Input: part model. Units: mm. Frame: model coordinates. Face numbers are marked on the shaded views. A direction names the side the tool comes from. Round coordinates to 2 decimals unless told otherwise and drop trailing zeros. Loops run counter-clockwise (first coordinate to the right, second up) from the corner with the lowest first, then second, coordinate; pieces in that order, holes last. Notation, with made-up numbers: (21, 44) -> (44, 44) arc R24 ccw to (44, 58) -> close; hole circle Ø2 at (18.25, -11.75). An arc over 180 degrees is marked (long way). One line per question, with ' | ' between items. Start each with the question number.
Q1. Material intervals for L1, parallel to X at y = 1.1, z = 0; L2, parallel to X at y = 2.75, z = -2.5; L3, parallel to Z at x = 0, y = 0.95, sorted ascending.
Q2. Cut plane C-C on x = 12.5. Return loops of the section in (y, z) (3 decimals), and give its area (3 significant figures).
Q3. Contact query for flat-ended pins moving along their axis: P1, Ø0.8, axis at x = 14, z = 0, coming from the +Y side; P2, Ø5, axis at x = 11.6, z = 0, coming from the -Y side; P3, Ø3.5, axis at y = 2, z = 2, coming from the -X side; P4, Ø6, axis at x = 0.5, z = -1.5, coming from the -Y side. Output: stop coordinate, or through.
Q4. Mould query, pull axis X, two halves, no side actions, for the marked faces 1, 2, 3 and 4. Classes: pulls with the +X half, pulls with the -X half, needs draft (parallel to the pull), parting line crosses it, or undercut.
Q5. Access query for the marked faces 5, 6 and 7. Directions: +Z, -Z, +X, -X, +Y, -Y. A direction counts if a zero-diameter tool reaches every point of the face in a straight line with its end or side. Return the directions, or none.
Q6. Cut plane B-B on z = 0. Return loops of the section in (x, y).
Q7. Cut plane A-A on y = 0.75. Return loops of the section in (x, z), and give its area (3 significant figures).
Q8. Cut plane D-D on z = 3.25. Return loops of the section in (x, y).
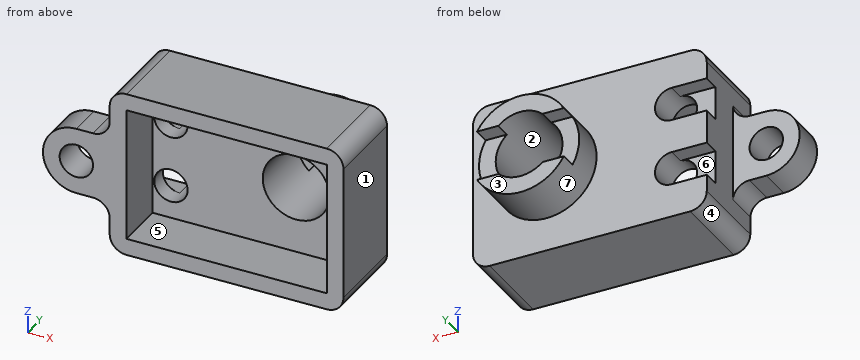
from build123d import *

# Parameters (mm, degrees)
SKETCH1_R           = 1
BOSS_EXTRUDE1_DEPTH = 5
SKETCH3_W           = 12
SKETCH3_H           = 8
CUT_EXTRUDE1_DEPTH  = 3
SKETCH4_R           = 3
SKETCH4_R_2         = 2
BOSS_EXTRUDE2_DEPTH = 3
SKETCH5_W           = 3
SKETCH5_H           = 1
CUT_EXTRUDE2_DEPTH  = 17
SKETCH6_R           = 2
SKETCH6_R_2         = 1
SKETCH6_W           = 7.064198251
SKETCH6_H           = 8.717344461
CUT_EXTRUDE3_DEPTH  = 6
CUT_EXTRUDE4_DEPTH  = 1


with BuildPart() as part:
    # Sketch1 → Boss-Extrude1 (new body)
    with BuildSketch(Plane(origin=(0, 0, 0), x_dir=(1, 0, 0), z_dir=(0, 1, 0))):
        with BuildLine():
            Line((1, 2), (0, 2))
            ThreePointArc((0, 2), (-2, 0), (0, -2))
            Line((0, -2), (1, -2))
            ThreePointArc((1, -2), (1.684527719, -2.270177533), (2, -2.935046948))
            Line((2, -2.935046948), (2, -4))
            ThreePointArc((2, -4), (2.292893219, -4.707106781), (3, -5))
            Line((3, -5), (15, -5))
            ThreePointArc((15, -5), (15.707106781, -4.707106781), (16, -4))
            Line((16, -4), (16, 4))
            ThreePointArc((16, 4), (15.707106781, 4.707106781), (15, 5))
            Line((15, 5), (3, 5))
            ThreePointArc((3, 5), (2.292893219, 4.707106781), (2, 4))
            Line((2, 4), (2, 2.932864189))
            ThreePointArc((2, 2.932864189), (1.684390871, 2.268771092), (1, 2))
        make_face()
        Circle(SKETCH1_R, mode=Mode.SUBTRACT)
    extrude(amount=BOSS_EXTRUDE1_DEPTH)

    # Sketch3 → Cut-Extrude1 (cut)
    with BuildSketch(Plane.XZ):
        with Locations((9, 0)):
            Rectangle(SKETCH3_W, SKETCH3_H)
    extrude(amount=-CUT_EXTRUDE1_DEPTH, mode=Mode.SUBTRACT)

    # Sketch4 → Boss-Extrude2 (add)
    with BuildSketch(Plane(origin=(0, 5, 0), x_dir=(1, 0, 0), z_dir=(0, 1, 0))):
        with Locations((11.597924937, 0)):
            Circle(SKETCH4_R)
        with Locations((11.597924937, 0)):
            Circle(SKETCH4_R_2, mode=Mode.SUBTRACT)
    extrude(amount=BOSS_EXTRUDE2_DEPTH)

    # Sketch5 → Cut-Extrude2 (cut)
    with BuildSketch(Plane.ZY.offset(-2)):
        with Locations((0, 7.5)):
            Rectangle(SKETCH5_W, SKETCH5_H)
    extrude(amount=-CUT_EXTRUDE2_DEPTH, mode=Mode.SUBTRACT)

    # Sketch6 → Cut-Extrude3 (cut)
    with BuildSketch(Plane(origin=(0, 8, 0), x_dir=(1, 0, 0), z_dir=(0, 1, 0))):
        with Locations((11.597924937, 0)):
            Circle(SKETCH6_R)
        with Locations((4.102933475, -2)):
            Circle(SKETCH6_R_2)
        with Locations((4.102933475, 2)):
            Circle(SKETCH6_R_2)
        with Locations((-1.532099126, -1.425808042)):
            Rectangle(SKETCH6_W, SKETCH6_H)
    extrude(amount=-CUT_EXTRUDE3_DEPTH, mode=Mode.SUBTRACT)

    # Sketch7 → Cut-Extrude4 (cut)
    with BuildSketch(Plane(origin=(0, 5, 0), x_dir=(1, 0, 0), z_dir=(0, 1, 0))):
        with BuildLine():
            Line((4.102933475, -3), (0.252638608, -3))
            ThreePointArc((0.252638608, -3), (-0.747361392, -2), (0.252638608, -1))
            Line((0.252638608, -1), (4.102933475, -1))
            ThreePointArc((4.102933475, -1), (5.102933475, -2), (4.102933475, -3))
        make_face()
        with BuildLine():
            Line((4.102933475, 1), (0.944196424, 1))
            ThreePointArc((0.944196424, 1), (-0.055803576, 2), (0.944196424, 3))
            Line((0.944196424, 3), (4.102933475, 3))
            ThreePointArc((4.102933475, 3), (5.102933475, 2), (4.102933475, 1))
        make_face()
    extrude(amount=-CUT_EXTRUDE4_DEPTH, mode=Mode.SUBTRACT)


solid = part.part
Results:
1) L1: -2 to -1, 1 to 3, 15 to 16 | L2: 2 to 3, 15 to 16 | L3: -2 to -1, 1 to 2
2) outline: (0, -5) -> (5, -5) -> (5, -2.861) -> (8, -2.861) -> (8, -1.785) -> (3, -1.785) -> (3, -4) -> (0, -4) -> close; (0, 4) -> (3, 4) -> (3, 1.785) -> (8, 1.785) -> (8, 2.861) -> (5, 2.861) -> (5, 5) -> (0, 5) -> close | area: 25.3 mm^2
3) P1: y = 7 | P2: y = 3 | P3: x = -1.98 | P4: y = 0
4) face 1: pulls with the +X half | face 2: undercut | face 3: needs draft | face 4: pulls with the -X half
5) face 5: -Y | face 6: -X, +Y | face 7: +Y
6) outline: (-2, 0) -> (-1, 0) -> (-1, 2) -> (-2, 2) -> close; (1, 0) -> (3, 0) -> (3, 3) -> (9.6, 3) -> (9.6, 7) -> (8.6, 7) -> (8.6, 5) -> (2, 5) -> (2, 2) -> (1, 2) -> close; (13.6, 3) -> (15, 3) -> (15, 0) -> (16, 0) -> (16, 5) -> (14.6, 5) -> (14.6, 7) -> (13.6, 7) -> close
7) outline: (0, -2) -> (1, -2) arc R1 cw to (2, -2.93) -> (2, -4) arc R1 ccw to (3, -5) -> (15, -5) arc R1 ccw to (16, -4) -> (16, 4) arc R1 ccw to (15, 5) -> (3, 5) arc R1 ccw to (2, 4) -> (2, 2.94) arc R1 cw to (1, 2) -> (0, 2) arc R2 ccw to start; hole circle Ø2 at (0, 0); hole (3, -4) -> (15, -4) -> (15, 4) -> (3, 4) -> close | area: 54.7 mm^2
8) outline: (2, 0) -> (3, 0) -> (3, 3) -> (15, 3) -> (15, 0) -> (16, 0) -> (16, 5) -> (2, 5) -> close
